```python
from build123d import *

# Parameters (mm, degrees)
ESQUISSE1_R             = 21.5
ESQUISSE1_R_2           = 20.5
BOSS_EXTRU_1_DEPTH      = 107
ESQUISSE2_R             = 20.5
ESQUISSE2_R_2           = 3
BOSS_EXTRU_2_DEPTH      = 5.5
CHANFREIN1_SIZE         = 2
CONG_1_R                = 10
ESQUISSE4_R             = 21.5
ESQUISSE4_R_2           = 20.5
ENL_V_MAT_EXTRU_2_DEPTH = 105


with BuildPart() as part:
    # Esquisse1 → Boss.-Extru.1 (new body)
    with BuildSketch(Plane(origin=(0, 0, 0), x_dir=(0, 0, -1), z_dir=(1, 0, 0))):
        Circle(ESQUISSE1_R)
        Circle(ESQUISSE1_R_2, mode=Mode.SUBTRACT)
    extrude(amount=BOSS_EXTRU_1_DEPTH)

    # Esquisse2 → Boss.-Extru.2 (add)
    with BuildSketch(Plane(origin=(107, 0, 0), x_dir=(0, 0, -1), z_dir=(1, 0, 0))):
        with BuildLine():
            ThreePointArc((6.205859778, 35.968559944), (14.711152146, 40.405222466), (18.372871483, 31.538668226))
            ThreePointArc((18.372871483, 31.538668226), (20.689295332, 23.844460332), (24.771129004, 16.923095695))
            ThreePointArc((24.771129004, 16.923095695), (28.662988941, 8.856244404), (30, 0))
            ThreePointArc((30, 0), (31.244976727, -6.50402438), (34.345135803, -12.355632184))
            ThreePointArc((34.345135803, -12.355632184), (37.237952026, -21.501974999), (27.870359387, -23.568900433))
            ThreePointArc((27.870359387, -23.568900433), (19.545131967, -25.015822985), (11.531193363, -27.69533498))
            ThreePointArc((11.531193363, -27.69533498), (5.879623738, -29.41819207), (0, -30))
            ThreePointArc((0, -30), (-9.148577813, -29.937932347), (-18.130212507, -31.678784611))
            ThreePointArc((-18.130212507, -31.678784611), (-27.639867217, -32.939911054), (-28.049234329, -23.355737059))
            ThreePointArc((-28.049234329, -23.355737059), (-26.447464851, -17.632677908), (-27.582285912, -11.799046736))
            ThreePointArc((-27.582285912, -11.799046736), (-26.28171566, 14.466216574), (-4.786405344, 29.615710761))
            ThreePointArc((-4.786405344, 29.615710761), (1.280514923, 31.804507658), (6.205859778, 35.968559944))
        make_face()
        Circle(ESQUISSE2_R, mode=Mode.SUBTRACT)
        with Locations((-23.461747754, -27.960622174)):
            Circle(ESQUISSE2_R_2, mode=Mode.SUBTRACT)
        with Locations((31.608959278, -18.251676453)):
            Circle(ESQUISSE2_R_2, mode=Mode.SUBTRACT)
        with Locations((12.487373333, 34.29745628)):
            Circle(ESQUISSE2_R_2, mode=Mode.SUBTRACT)
        with BuildLine():
            ThreePointArc((-26.420087149, 5.268613512), (-26.8090472, 2.647058824), (-26.939118291, 0))
            ThreePointArc((-26.939118291, 0), (-25.439118291, -1.5), (-23.939118291, 0))
            ThreePointArc((-23.939118291, 0), (-23.823499543, 2.352941176), (-23.477757276, 4.68321201))
            ThreePointArc((-23.477757276, 4.68321201), (-24.656221462, 6.447077698), (-26.420087149, 5.268613512))
        make_face(mode=Mode.SUBTRACT)
        with BuildLine():
            ThreePointArc((5.329495221, 26.480968858), (2.707940533, 26.869928909), (0.060881709, 27))
            ThreePointArc((0.060881709, 27), (-1.439118291, 25.5), (0.060881709, 24))
            ThreePointArc((0.060881709, 24), (2.413822886, 23.884381253), (4.74409372, 23.538638985))
            ThreePointArc((4.74409372, 23.538638985), (6.507959407, 24.717103171), (5.329495221, 26.480968858))
        make_face(mode=Mode.SUBTRACT)
        with BuildLine():
            ThreePointArc((26.541850567, -5.268613512), (26.930810618, -2.647058824), (27.060881709, 0))
            ThreePointArc((27.060881709, 0), (25.560881709, 1.5), (24.060881709, 0))
            ThreePointArc((24.060881709, 0), (23.945262962, -2.352941176), (23.599520694, -4.68321201))
            ThreePointArc((23.599520694, -4.68321201), (24.77798488, -6.447077698), (26.541850567, -5.268613512))
        make_face(mode=Mode.SUBTRACT)
        with BuildLine():
            ThreePointArc((-5.207731802, -26.480968858), (-2.586177114, -26.869928909), (0.060881709, -27))
            ThreePointArc((0.060881709, -27), (1.560881709, -25.5), (0.060881709, -24))
            ThreePointArc((0.060881709, -24), (-2.292059467, -23.884381253), (-4.622330301, -23.538638985))
            ThreePointArc((-4.622330301, -23.538638985), (-6.386195988, -24.717103171), (-5.207731802, -26.480968858))
        make_face(mode=Mode.SUBTRACT)
    extrude(amount=-BOSS_EXTRU_2_DEPTH)

    # Chanfrein1
    chanfrein1_edges = [part.edges().sort_by_distance(p)[0] for p in [
        (107, 6.447077698, 24.656221462),
        (107, 2.352941176, 23.823499543),
        (107, -1.5, 25.439118291),
        (107, 2.647058824, 26.8090472),
        (107, 24.717103171, -6.507959407),
        (107, 23.884381253, -2.413822886),
        (107, 25.5, 1.439118291),
        (107, 26.869928909, -2.707940533),
        (107, -6.447077698, -24.77798488),
        (107, -2.352941176, -23.945262962),
        (107, 1.5, -25.560881709),
        (107, -2.647058824, -26.930810618),
        (107, -24.717103171, 6.386195988),
        (107, -23.884381253, 2.292059467),
        (107, -25.5, -1.560881709),
        (107, -26.869928909, 2.586177114),
    ]]
    chamfer(chanfrein1_edges, length=CHANFREIN1_SIZE)

    # Congé1
    cong_1_edges = [part.edges().sort_by_distance(p)[0] for p in [
        (104.25, 35.968559944, -6.205859778),
        (104.25, 31.538668226, -18.372871483),
        (104.25, -12.355632184, -34.345135803),
        (104.25, -23.568900433, -27.870359387),
        (104.25, -31.678784611, 18.130212507),
        (104.25, -23.355737059, 28.049234329),
    ]]
    fillet(cong_1_edges, radius=CONG_1_R)

    # Esquisse4 → Enlèv. mat.-Extru.2 (cut)
    with BuildSketch(Plane.ZY):
        Circle(ESQUISSE4_R)
        Circle(ESQUISSE4_R_2, mode=Mode.SUBTRACT)
    extrude(amount=-ENL_V_MAT_EXTRU_2_DEPTH, mode=Mode.SUBTRACT)


solid = part.part
```
Here's how the part is built. I have some questions about the finished solid (model axes, mm). A direction names the side the tool comes from. Give positions to 0.01 mm unless a question says otherwise; leave off trailing zeros. Write each loop counter-clockwise with the first axis right and the second up, starting at its lowest first coordinate (ties: lowest second). Pieces come first, ordered by that corner, then holes. Notation, with made-up numbers: M 37.25,78 L 51.25,78 A9 cw 51.25,84 Z; hole C 19.25,60.25 d11. An arc over 180 degrees is marked long. Put each result on its own line as item: value. Start each with the question number.
Item 1: I need wall thicknesses on L1, parallel to Z at x = 103, y = 0; L2, parallel to Y at x = 106.65, z = -13; L3, parallel to Z at x = 106.2, y = 6. Which ranges of each line are inside material? Lowest first, please. Write a range as from..to.
Item 2: On a 3-axis mill with a long thin cutter (end or side, diameter ignored), from which of +Z, -Z, +X, -X, +Y, -Y can I reach the whole of each face in a straight line? I mean faces 1 (the cylindrical face through (103.274, 2.32, 23.827)), 2 (the cylindrical face through (103.226, 21.317, -2.799)), 3 (the cylindrical face through (104.3, -25.4, -18.1)). Say none if no direction works.
Item 3: Will these pins go through, and if not, where does the flat tip stop? pin 1 (2 mm diameter, centred on x = 103.5, z = -23.5, fed in from -Y); pin 2 (1 mm diameter, centred on x = 104, z = -4.5, fed in from +Y); pin 3 (3 mm diameter, centred on x = 103.5, z = 15.5, fed in from -Y).
Item 4: If we section it at B-B, the plane z = -2.5: Count the separate pieces of the cut face and the enclosed holes in it, then the cut area to 3 significant figures.
Item 5: If we section it at A-A, the plane z = 12: Write out the boundary of the cut face in (x, y), then the cut area to 3 significant figures.
Item 6: Thinking about a two-plate mould opening in Y: for faces 4 (the cylindrical face through (104.288, -29.814, 7.487)), 5 (the cylindrical face through (103.27, -2.32, -23.95)), 6 (the cylindrical face through (104.288, -5.041, -30.786)), which applies, +Y half, -Y half, draft (parallel to the pull), parting line (faces both ways), or undercut?
Values:
1. L1: -30..-27.06, -24.06..-21.5, 21.5..23.94, 26.94..30
1. L2: -27.1..-15.85, 15.85..31.34, 37.25..40.78
1. L3: -29.39..-19.6, 19.6..22.45, 27.45..29.39
2. face 1: +X, -X
2. face 2: -X
2. face 3: +X, -X, -Y
3. pin 1: y = -24.35
3. pin 2: y = 34.69
3. pin 3: y = -31.52
4. separate pieces: 3
4. enclosed holes: 0
4. area: 88.7 mm²
5. outline: M 101.5,-30.29 L 107,-30.29 L 107,-16.62 L 105,-16.62 L 105,-17.84 L 101.5,-17.84 Z; M 101.5,17.84 L 105,17.84 L 105,16.62 L 107,16.62 L 107,27.5 L 101.5,27.5 Z
5. area: 126 mm²
6. face 4: -Y half
6. face 5: undercut
6. face 6: +Y half
